Build history of the part. All positions in model axes, mm. Face numbers are marked on the shaded views. A direction names the side the tool comes from. Round coordinates to 2 decimals unless told otherwise and drop trailing zeros. Write each loop counter-clockwise with the first axis right and the second up, starting at its lowest first coordinate (ties: lowest second). Pieces come first, ordered by that corner, then holes. Notation, with made-up numbers: (24, 53) -> (64, 53) arc R37 cw to (64, 89) -> close; hole circle Ø4 at (15, 73). An arc over 180 degrees is marked (long way). Answer in a Markdown table with one row per item. Add a question column.
from build123d import *

# Parameters (mm, degrees)
EXTRUDE_1_DEPTH = 2
SKETCH_1_6_W    = 2
SKETCH_1_6_H    = 4
SKETCH_1_6_W_2  = 4
SKETCH_1_6_H_2  = 1.5
EXTRUDE_2_DEPTH = 7.5
EXTRUDE_START   = 7.5
SKETCH_1_7_W    = 3
SKETCH_1_7_H    = 4
SKETCH_1_7_R    = 0.6
EXTRUDE_3_DEPTH = 1.5


with BuildPart() as part:
    # 草图1 → 凸台-拉伸1 (new body)
    with BuildSketch(Plane.XY):
        Polygon((-2, 4), (-2, -4), (-14.6, -4), (-14.6, -8), (14.6, -8), (14.6, -4), (2, -4), (2, 4), (14.6, 4), (14.6, 8), (-14.6, 8), (-14.6, 4), align=None)
    extrude(amount=EXTRUDE_1_DEPTH)

    # 草图1<6> → 凸台-拉伸2 (add)
    with BuildSketch(Plane.XY):
        with Locations((15.6, -6)):
            Rectangle(SKETCH_1_6_W, SKETCH_1_6_H)
        with Locations((15.6, 6)):
            Rectangle(SKETCH_1_6_W, SKETCH_1_6_H)
        with Locations((-15.6, 6)):
            Rectangle(SKETCH_1_6_W, SKETCH_1_6_H)
        with Locations((-15.6, -6)):
            Rectangle(SKETCH_1_6_W, SKETCH_1_6_H)
        with Locations((0, 0.75)):
            Rectangle(SKETCH_1_6_W_2, SKETCH_1_6_H_2)
        with Locations((0, -0.75)):
            Rectangle(SKETCH_1_6_W_2, SKETCH_1_6_H_2)
    extrude(amount=EXTRUDE_2_DEPTH)

    # 草图1<7> → 凸台-拉伸3 (add)
    # profile 1 of 6: a face of its own
    with BuildSketch(Plane.XY.offset(EXTRUDE_START)):
        with Locations((18.1, 6)):
            Rectangle(SKETCH_1_7_W, SKETCH_1_7_H)
        with Locations((18.1, 6)):
            Circle(SKETCH_1_7_R, mode=Mode.SUBTRACT)
    # profile 2 of 6: a face of its own
    with BuildSketch(Plane.XY.offset(EXTRUDE_START)):
        with Locations((18.1, -6)):
            Rectangle(SKETCH_1_7_W, SKETCH_1_7_H)
        with Locations((18.1, -6)):
            Circle(SKETCH_1_7_R, mode=Mode.SUBTRACT)
    # profile 3 of 6: a face of its own
    with BuildSketch(Plane.XY.offset(EXTRUDE_START)):
        with Locations((-18.1, 6)):
            Rectangle(SKETCH_1_7_W, SKETCH_1_7_H)
        with Locations((-18.1, 6)):
            Circle(SKETCH_1_7_R, mode=Mode.SUBTRACT)
    # profile 4 of 6: a face of its own
    with BuildSketch(Plane.XY.offset(EXTRUDE_START)):
        with Locations((-18.1, -6)):
            Rectangle(SKETCH_1_7_W, SKETCH_1_7_H)
        with Locations((-18.1, -6)):
            Circle(SKETCH_1_7_R, mode=Mode.SUBTRACT)
    # profile 5 of 6: a face of its own
    with BuildSketch(Plane.XY.offset(EXTRUDE_START)):
        Polygon((-2, -1.5), (-2, 0), (-2, 1.5), (-5, 1.5), (-5, -1.5), align=None)
        with Locations((-3.5, 0)):
            Circle(SKETCH_1_7_R, mode=Mode.SUBTRACT)
    # profile 6 of 6: a face of its own
    with BuildSketch(Plane.XY.offset(EXTRUDE_START)):
        Polygon((2, 1.5), (2, 0), (2, -1.5), (5, -1.5), (5, 1.5), align=None)
        with Locations((3.5, 0)):
            Circle(SKETCH_1_7_R, mode=Mode.SUBTRACT)
    extrude(amount=-EXTRUDE_3_DEPTH)


solid = part.part
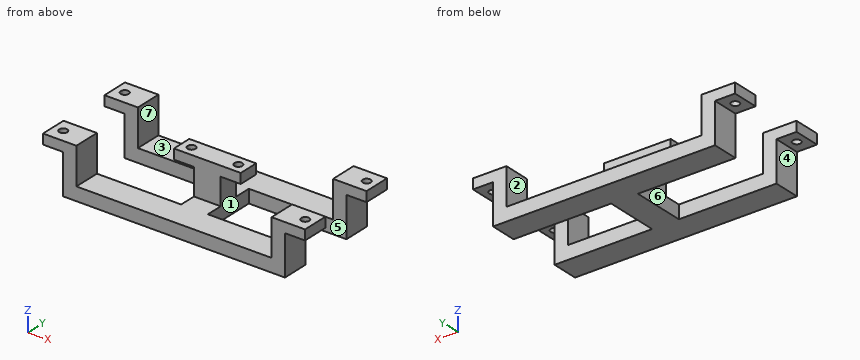
(1) Saw through at D-D (x = 18.1). List the corners of the cut face in (y, z).
(2) Saw through at A-A (y = -6). List the corners of the cut face in (x, z).
(3) Saw through at B-B (x = -12). List the corners of the cut face in (y, z), plus the area to 3 significant figures.
(4) Probe line 1 along Y through (x, z) = (-18.1, 6.95); line 2 along X through (y, z) = (-6.5, 3.25); line 3 along Y through (x, z) = (12, 1.5). List the from-to ranges inside material, lowest first.
(5) Drop flat-ended pins along their axis: P1, Ø1.5, axis at x = 18.5, y = 5, coming from the -Z side; P2, Ø1, axis at x = 18.1, y = 6, coming from the +Z side; P3, Ø3, axis at x = -5.5, y = 6, coming from the +Z side; P4, Ø2, axis at y = 6, z = 4.5, coming from the +X side. Give the stop position or say it passes through.
(6) Mould opens along X. For the marked faces 5, 6 and 7 say: pulls with the +X half, pulls with the -X half, needs draft (parallel to the pull), parting line crosses it, or undercut.
(7) Which spindle directions (+Z, -Z, +X, -X, +Y, -Y) get a long thin tool onto all of the face, cutting with end or side? Do the marked faces 1, 2, 3 and 4. Say none if no direction does.
(8) Saw through at C-C (z = 5.5). List the corners of the cut face in (x, y), plus the area to 3 significant figures.
Answer sheet:
| question | item | result |
|---|---|---|
| 1 | outline | (-8, 6) -> (-6.6, 6) -> (-6.6, 7.5) -> (-8, 7.5) -> close; (-5.4, 6) -> (-4, 6) -> (-4, 7.5) -> (-5.4, 7.5) -> close; (4, 6) -> (5.4, 6) -> (5.4, 7.5) -> (4, 7.5) -> close; (6.6, 6) -> (8, 6) -> (8, 7.5) -> (6.6, 7.5) -> close |
| 2 | outline | (-19.6, 6) -> (-18.7, 6) -> (-18.7, 7.5) -> (-19.6, 7.5) -> close; (-17.5, 6) -> (-16.6, 6) -> (-16.6, 0) -> (16.6, 0) -> (16.6, 6) -> (17.5, 6) -> (17.5, 7.5) -> (14.6, 7.5) -> (14.6, 2) -> (-14.6, 2) -> (-14.6, 7.5) -> (-17.5, 7.5) -> close; (18.7, 6) -> (19.6, 6) -> (19.6, 7.5) -> (18.7, 7.5) -> close |
| 3 | outline | (-8, 0) -> (-4, 0) -> (-4, 2) -> (-8, 2) -> close; (4, 0) -> (8, 0) -> (8, 2) -> (4, 2) -> close |
| 3 | area | 16.0 mm² |
| 4 | line 1 | y = -8 to -6.6, -5.4 to -4, 4 to 5.4, 6.6 to 8 |
| 4 | line 2 | x = -16.6 to -14.6, 14.6 to 16.6 |
| 4 | line 3 | y = -8 to -4, 4 to 8 |
| 5 | P1 | stops at z = 6 |
| 5 | P2 | passes through |
| 5 | P3 | stops at z = 2 |
| 5 | P4 | stops at x = 16.6 |
| 6 | face 5 | needs draft |
| 6 | face 6 | pulls with the -X half |
| 6 | face 7 | undercut |
| 7 | face 1 | -Z, +X |
| 7 | face 2 | +Z, +Y, -Y |
| 7 | face 3 | +Z, +Y |
| 7 | face 4 | -Z, -X, +Y, -Y |
| 8 | outline | (-16.6, -8) -> (-14.6, -8) -> (-14.6, -4) -> (-16.6, -4) -> close; (-16.6, 4) -> (-14.6, 4) -> (-14.6, 8) -> (-16.6, 8) -> close; (-2, -1.5) -> (2, -1.5) -> (2, 1.5) -> (-2, 1.5) -> close; (14.6, -8) -> (16.6, -8) -> (16.6, -4) -> (14.6, -4) -> close; (14.6, 4) -> (16.6, 4) -> (16.6, 8) -> (14.6, 8) -> close |
| 8 | area | 44.0 mm² |
